Design review of the part built by this model. Coordinates are the model's own, in mm. Give positions to 0.01 mm unless a question says otherwise; leave off trailing zeros. Loops run counter-clockwise (first coordinate to the right, second up) from the corner with the lowest first, then second, coordinate; pieces in that order, holes last.
Autodesk Inventor part; units mm, degrees
ref_plane "YZ Plane" through (0, 0, 0) normal (1, 0, 0) x (0, 1, 0)
ref_plane "XZ Plane" through (0, 0, 0) normal (0, 1, 0) x (-1, 0, 0)
ref_plane "XY Plane" through (0, 0, 0) normal (0, 0, 1) x (1, 0, 0)
sketch "Sketch1" plane through (0, 0, 0) normal (0, 0, 1) x (1, 0, 0)
  line L0 (-63.5, -63.5) -> (63.5, -63.5)
  line L1 (63.5, -63.5) -> (63.5, 63.5)
  line L2 (63.5, 63.5) -> (-63.5, 63.5)
  line L3 (-63.5, 63.5) -> (-63.5, -63.5)
  point P0 (0, 0)
  dimension "d19" = 63.5
extrude "Extrusion1" add sketch "Sketch1" against normal blind 6.35
sketch "Sketch2" plane through (0, 0, 0) normal (0, 0, 1) x (1, 0, 0)
  circle A0 centre (-25.4, 38.1) radius 12.7
  line L0 (63.5, 63.5) -> (-63.5, 63.5)
  line L1 (-63.5, -63.5) -> (-63.5, 63.5)
  dimension "d4" = 25.4
  dimension "d20" = 25.4
  dimension "d23" = 38.1
extrude "Extrusion2" cut sketch "Sketch2" against normal through all
sketch "Sketch3" plane through (0, 0, 0) normal (0, 0, 1) x (1, 0, 0)
  circle A0 centre (-25.4, 38.1) radius 23.8125 construction
  line L0 (63.5, 63.5) -> (-63.5, 63.5)
  line L1 (-63.5, 63.5) -> (-63.5, -63.5)
  point P0 (-15.0599, 59.5503)
  point P1 (-1.6534, 39.8703)
  point P2 (-11.9935, 18.42)
  point P3 (-35.7401, 16.6497)
  point P4 (-49.1466, 36.3297)
  point P5 (-38.8065, 57.78)
  dimension "d7" = 47.625
  dimension "d10" = 360
  dimension "d21" = 25.4
  dimension "d22" = 38.1
hole "Hole1" at (-15.0599, 59.5503, 0) at (-1.6534, 39.8703, 0) at (-11.9935, 18.42, 0) at (-35.7401, 16.6497, 0) at (-49.1466, 36.3297, 0) at (-38.8065, 57.78, 0) direction (0, 0, -1) diameter 5.1054 end through all
properties part number "supportPlateForLinearActuator"
Q1. Insertion check: pin 1 (6 mm diameter, centred on x = -15.06, y = 59.55, fed in from -Z); pin 2 (4.5 mm diameter, centred on x = -11.99, y = 18.42, fed in from +Z). Each pin has a flat end and moves straight along its axis. Give the tip position at first contact, or say it passes through.
Results:
pin 1: stops at z = -6.35
pin 2: passes through
Q2. Take a section at A-A (x = -25.4). Give the boundary of the cut face in (y, z).
Results:
outline: (-63.5, -6.35) - (25.4, -6.35) - (25.4, 0) - (-63.5, 0) - close; (50.8, -6.35) - (63.5, -6.35) - (63.5, 0) - (50.8, 0) - close
Q3. Wall thickness on line 1 (Y direction, x = -14, z = -0.5); line 2 (X direction, y = 18.42, z = -2.75); line 3 (Y direction, x = -25.5, z = -2.25): over which ranges is each line inside the solid? List them lowest first.
Results:
line 1: y = -63.5 to 16.84, 20 to 32.5, 43.7 to 57.23, 61.87 to 63.5
line 2: x = -63.5 to -37.58, -33.9 to -14.55, -9.44 to 63.5
line 3: y = -63.5 to 25.4, 50.8 to 63.5
Q4. Take a section at B-B (z = -1.25). Give the boundary of the cut face in (x, y), plus the area to 3 significant figures.
Results:
outline: (-63.5, -63.5) - (63.5, -63.5) - (63.5, 63.5) - (-63.5, 63.5) - close; hole circle Ø5.11 at (-49.15, 36.33); hole circle Ø5.11 at (-38.81, 57.78); hole circle Ø5.11 at (-35.74, 16.65); hole circle Ø25.4 at (-25.4, 38.1); hole circle Ø5.11 at (-15.06, 59.55); hole circle Ø5.11 at (-11.99, 18.42); hole circle Ø5.11 at (-1.65, 39.87)
area: 15,500 mm2
Q5. Draft analysis for pull direction X (two halves, no side actions). For faces 1 (the face through (-14, 20, -3)), 2 (the face through (-1, 1, -6.35)), 3 (the face through (-63.5, 1, -3)), state which applies: pulls with the +X half, pulls with the -X half, needs draft (parallel to the pull), parting line crosses it, or undercut.
Results:
face 1: undercut
face 2: needs draft
face 3: pulls with the -X half
